from build123d import *

# Parameters (mm, degrees)
F1_DEPTH = 2.5


with BuildPart() as f1:
    # F0 (on Front) → F1 (new body, symmetric)
    with BuildSketch(Plane.XZ):
        with BuildLine():
            Line((5, -20), (5, 0))
            Line((5, 0), (2.5, 0))
            ThreePointArc((2.5, 0), (0, -2.5), (-2.5, 0))
            Line((-2.5, 0), (-5, 0))
            Line((-5, 0), (-5, -20))
            Line((-5, -20), (5, -20))
        make_face()
        with BuildLine():
            Line((2.5, 0), (5, 0))
            ThreePointArc((5, 0), (0, 5), (-5, 0))
            Line((-5, 0), (-2.5, 0))
            ThreePointArc((-2.5, 0), (0, 2.5), (2.5, 0))
        make_face()
    extrude(amount=F1_DEPTH, both=True)


solid = f1.part
The listing builds one solid part. Answer for the finished solid, in the listing's coordinates (mm). Coordinates: 2 decimals unless noted, no trailing zeros. Write each loop counter-clockwise with the first axis right and the second up, starting at its lowest first coordinate (ties: lowest second). Pieces come first, ordered by that corner, then holes. Notation, with made-up numbers: (-22, 53.5) - (-16, 53.5) arc R26 cw to (-16, 68.5) - close; hole circle Ø11 at (21, 59). An arc over 180 degrees is marked (long way). Put each result on its own line as item: value.
1. The part is cut by section D-D on x = 3.25. Give the vertices of the cut face in (y, z), plus the area to 3 significant figures.
Answer sheet:
outline: (-2.5, -20) - (2.5, -20) - (2.5, 3.8) - (-2.5, 3.8) - close
area: 119 mm^2
2. Determine the mould class of faces 1 (the face through (2, 0, -1.5)), 2 (the face through (0, 0, 5)), 3 (the face through (0, -2.5, -7)), 4 (the face through (0, 0, -20)) for opening direction Z: pulls with the +Z half, pulls with the -Z half, needs draft (parallel to the pull), parting line crosses it, or undercut.
Answer sheet:
face 1: undercut
face 2: pulls with the +Z half
face 3: needs draft
face 4: pulls with the -Z half
3. The part is cut by section A-A on x = 0. Give the vertices of the cut face in (y, z).
Answer sheet:
outline: (-2.5, -20) - (2.5, -20) - (2.5, -2.5) - (-2.5, -2.5) - close; (-2.5, 2.5) - (2.5, 2.5) - (2.5, 5) - (-2.5, 5) - close
4. Flat-ended cylindrical pins translate along their axes: pin 1 Ø1 at (y, z) = (-1.5, 2) entering from -X; pin 2 Ø1 at (x, y) = (-4, 0.5) entering from +Z; pin 3 Ø4 at (x, z) = (0, 0) entering from +Y. Find the tip coordinate at first contact, or state that the pin passes through.
Answer sheet:
pin 1: stops at x = -4.77
pin 2: stops at z = 3.57
pin 3: passes through
5. The part is cut by section C-C on z = 1. Give the vertices of the cut face in (x, y), plus the area to 3 significant figures.
Answer sheet:
outline: (-4.9, -2.5) - (-2.29, -2.5) - (-2.29, 2.5) - (-4.9, 2.5) - close; (2.29, -2.5) - (4.9, -2.5) - (4.9, 2.5) - (2.29, 2.5) - close
area: 26.1 mm^2
6. Find the intervals of material crossed by line 1 along Z through (x, y) = (0, -1.3); line 2 along Z through (x, y) = (-0.5, 1.45); line 3 along X through (y, z) = (-1.2, 2), in increasing order. Write a range as from..to.
Answer sheet:
line 1: z = -20..-2.5, 2.5..5
line 2: z = -20..-2.45, 2.45..4.97
line 3: x = -4.58..-1.5, 1.5..4.58
7. The part is cut by section B-B on y = -1.1. Give the vertices of the cut face in (x, z), plus the area to 3 significant figures.
Answer sheet:
outline: (-5, -20) - (5, -20) - (5, 0) arc R5 ccw to (-5, 0) - close; hole circle Ø5 at (0, 0)
area: 220 mm^2
